The figure shows three views and two pictorial views of one solid part (mm, origin at its lowest corner). Answer the questions. A direction names the side the tool comes from. Round coordinates to 2 decimals unless told otherwise and drop trailing zeros. Loops run counter-clockwise (first coordinate to the right, second up) from the corner with the lowest first, then second, coordinate; pieces in that order, holes last. Notation, with made-up numbers: (76.25, 23) -> (93.25, 23) arc R20 ccw to (93.25, 36) -> close; hole circle Ø1 at (-0.75, 27.5). An arc over 180 degrees is marked (long way). Use a Markdown table: item, result. Add a question column.
Q1. Which of the six approach directions +Z, -Z, +X, -X, +Y, -Y give full straight-line access (tool end or side, diameter ignored) to the marked faces 1 and 2?
Q2. Section C-C on y = 6 is taken. Give the vertices of the cut face in (x, z), then the cut area to 3 significant figures.
Q3. Given pin 1 Ø10 at (x, y) = (7.5, 4) entering from +Z; pin 2 Ø1.1 at (x, y) = (5, 0.5) entering from -Z; pin 3 Ø1.1 at (y, z) = (0.5, 18.5) entering from -X, each flat-ended and moving along its own axis, determine where each tip first touches the part or whether it passes through.
Q4. Consider line 1 (Y direction, x = 16.5, z = 8); line 2 (Z direction, x = 21.75, y = 18.5). Determine where each line is inside the solid, lowest interval first.
Q5. Section A-A on x = 18 is taken. Give the vertices of the cut face in (y, z), then the cut area to 3 significant figures.
Q6. Section B-B on z = 45 is taken. Give the vertices of the cut face in (x, y), then the cut area to 3 significant figures.
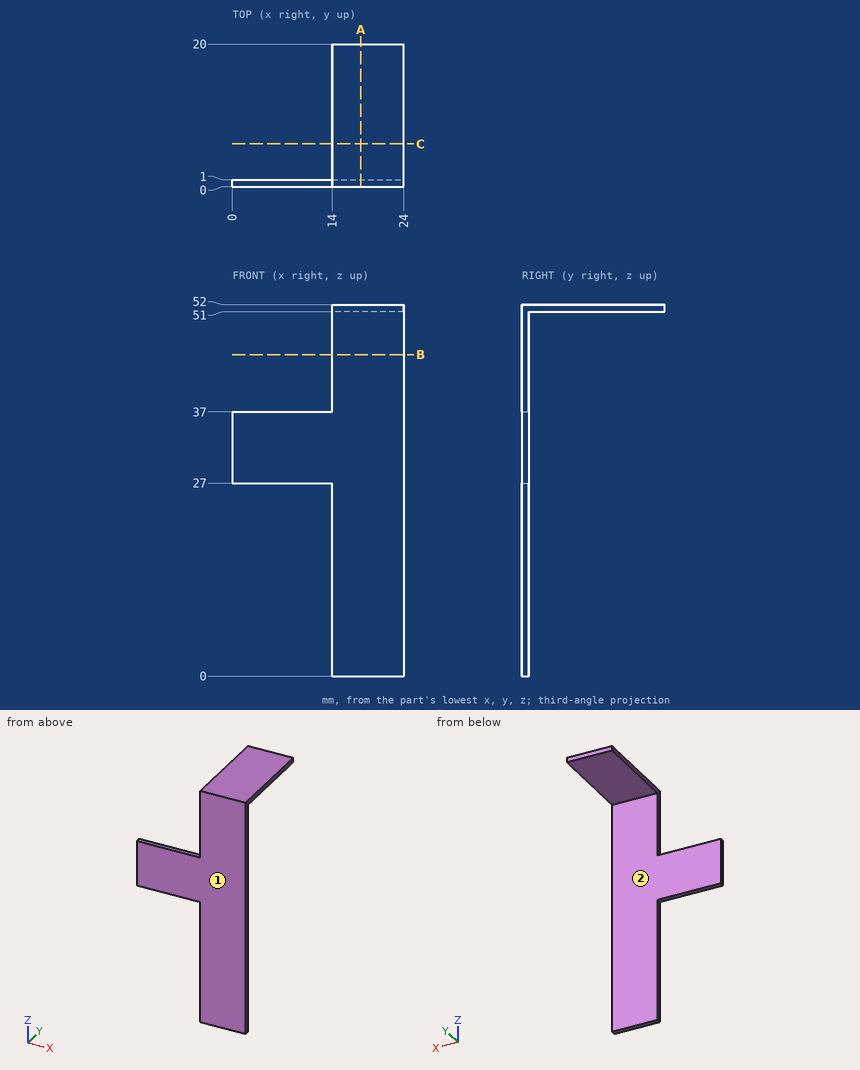
Checked values:
| question | item | result |
|---|---|---|
| 1 | face 1 | +Z, -Z, +X, -X, -Y |
| 1 | face 2 | -Z, +X, -X, +Y |
| 2 | outline | (14, 51) -> (24, 51) -> (24, 52) -> (14, 52) -> close |
| 2 | area | 10.0 mm2 |
| 3 | pin 1 | stops at z = 37 |
| 3 | pin 2 | stops at z = 27 |
| 3 | pin 3 | stops at x = 14 |
| 4 | line 1 | y = 0 to 1 |
| 4 | line 2 | z = 51 to 52 |
| 5 | outline | (0, 0) -> (1, 0) -> (1, 51) -> (20, 51) -> (20, 52) -> (0, 52) -> close |
| 5 | area | 71.0 mm2 |
| 6 | outline | (14, 0) -> (24, 0) -> (24, 1) -> (14, 1) -> close |
| 6 | area | 10.0 mm2 |
